from build123d import *

# Parameters (mm, degrees)
SKETCH1_W                = 36
SKETCH1_H                = 22.4
SKETCH1_R                = 1.6
BOSS_EXTRUDE1_DEPTH      = 9.35
FILLET1_R                = 5
SKETCH2_R                = 3.5
BOSS_EXTRUDE2_DEPTH      = 0.3
BOSS_EXTRUDE4_START      = -0.3
BOSS_EXTRUDE4_DEPTH      = 8.4
M3_CLEARANCE_HOLE1_D     = 3.4
M3_CLEARANCE_HOLE1_DEPTH = 8.0000094
M3_CLEARANCE_HOLE1_TIP   = 1.021463052
BOSS_EXTRUDE5_DEPTH      = 9.5
BOSS_EXTRUDE6_DEPTH      = 23
BOSS_EXTRUDE7_DEPTH      = 13.5
SKETCH11_W               = 3.9
SKETCH11_H               = 13.4
CUT_EXTRUDE1_DEPTH       = 5
SKETCH13_W               = 4.8
SKETCH13_H               = 5
SKETCH13_R               = 1.5
BOSS_EXTRUDE8_DEPTH      = 2.75
FILLET2_R                = 1


with BuildPart() as part:
    # Sketch1 → Boss-Extrude1 (new, symmetric)
    with BuildSketch(Plane(origin=(0, 0, 0), x_dir=(1, 0, 0), z_dir=(0, 1, 0))):
        Rectangle(SKETCH1_W, SKETCH1_H)
        with Locations(Location((-13, 8.75, 0), (0, 0, 270))):
            Circle(SKETCH1_R, mode=Mode.SUBTRACT)
        with Locations(Location((-13, -8.75, 0), (0, 0, 270))):
            Circle(SKETCH1_R, mode=Mode.SUBTRACT)
    extrude(amount=BOSS_EXTRUDE1_DEPTH, both=True)

    # Fillet1
    fillet1_edges = [part.edges().sort_by_distance(p)[0] for p in [
        (18, 0, 11.2),
        (18, 0, -11.2),
    ]]
    fillet(fillet1_edges, radius=FILLET1_R)

    # Sketch2 → Boss-Extrude2 (add)
    with BuildSketch(Plane(origin=(0, 9.35, 0), x_dir=(1, 0, 0), z_dir=(0, 1, 0))):
        with Locations(Location((6.7, 0, 0), (0, 0, 90))):
            Circle(SKETCH2_R)
    extrude(amount=BOSS_EXTRUDE2_DEPTH)

    # Sketch3 → Boss-Extrude4 (add)
    with BuildSketch(Plane(origin=(0, 9.65, 0), x_dir=(1, 0, 0), z_dir=(0, 1, 0)).offset(BOSS_EXTRUDE4_START)):
        with BuildLine():
            ThreePointArc((4.716700981, 1.905), (4.148865713, 1.026749165), (3.95, 0))
            Line((3.95, 0), (9.45, 0))
            ThreePointArc((9.45, 0), (9.251134287, 1.026749165), (8.683299019, 1.905))
            Line((8.683299019, 1.905), (4.716700981, 1.905))
        make_face()
        with BuildLine():
            Line((9.45, 0), (3.95, 0))
            ThreePointArc((3.95, 0), (4.148865713, -1.026749165), (4.716700981, -1.905))
            Line((4.716700981, -1.905), (8.683299019, -1.905))
            ThreePointArc((8.683299019, -1.905), (9.251134287, -1.026749165), (9.45, 0))
        make_face()
    extrude(amount=BOSS_EXTRUDE4_DEPTH)

    # M3 Clearance Hole1
    with Locations(Plane(origin=(6.7, 17.75, 0), x_dir=(0, 0, 1), z_dir=(0, 1, 0))):
        with Locations((0, 0)):
            Hole(M3_CLEARANCE_HOLE1_D / 2, depth=M3_CLEARANCE_HOLE1_DEPTH)
            with Locations((0, 0, -(M3_CLEARANCE_HOLE1_DEPTH + M3_CLEARANCE_HOLE1_TIP / 2))):  # 118° drill point
                Cone(0, M3_CLEARANCE_HOLE1_D / 2, M3_CLEARANCE_HOLE1_TIP, mode=Mode.SUBTRACT)

    # Sketch7 → Boss-Extrude5 (add)
    with BuildSketch(Plane.ZY.offset(18)):
        with BuildLine():
            ThreePointArc((-11.2, -2.901648127), (-10.306415682, -6.352188829), (-8.378242386, -9.35))
            Line((-8.378242386, -9.35), (8.378242386, -9.35))
            ThreePointArc((8.378242386, -9.35), (10.306415682, -6.352188829), (11.2, -2.901648127))
            Line((11.2, -2.901648127), (11.2, -0.782686117))
            ThreePointArc((11.2, -0.782686117), (9.493833141, 4.193529382), (5.711776998, 7.85))
            Line((5.711776998, 7.85), (-5.711776998, 7.85))
            ThreePointArc((-5.711776998, 7.85), (-9.493833141, 4.193529382), (-11.2, -0.782686117))
            Line((-11.2, -0.782686117), (-11.2, -2.901648127))
        make_face()
    extrude(amount=BOSS_EXTRUDE5_DEPTH)

    # Sketch8 → Boss-Extrude6 (add)
    with BuildSketch(Plane.ZY.offset(27.5)):
        with BuildLine():
            Line((12.7, -2.97021854), (12.7, -0.714115705))
            ThreePointArc((12.7, -0.714115705), (10.665331767, 5.144477158), (6.107200268, 9.35))
            Line((6.107200268, 9.35), (-6.107200268, 9.35))
            ThreePointArc((-6.107200268, 9.35), (-10.665331767, 5.144477158), (-12.7, -0.714115705))
            Line((-12.7, -0.714115705), (-12.7, -2.97021854))
            ThreePointArc((-12.7, -2.97021854), (-11.554180407, -7.233216661), (-9.023383337, -10.85))
            Line((-9.023383337, -10.85), (9.023383337, -10.85))
            ThreePointArc((9.023383337, -10.85), (11.554180407, -7.233216661), (12.7, -2.97021854))
        make_face()
    extrude(amount=BOSS_EXTRUDE6_DEPTH)

    # Sketch9 → Boss-Extrude7 (add)
    with BuildSketch(Plane.ZY.offset(57.000000114)):
        with BuildLine():
            Line((-8.4, -1.842167122), (-8.4, -6.489747138))
            ThreePointArc((-8.4, -6.489747138), (0, -11.442167122), (8.4, -6.489747138))
            Line((8.4, -6.489747138), (8.4, -1.842167122))
            Line((8.4, -1.842167122), (-8.4, -1.842167122))
        make_face()
        with BuildLine():
            ThreePointArc((8.4, -6.489747138), (0, -11.442167122), (-8.4, -6.489747138))
            Line((-8.4, -6.489747138), (-8.4, -18.454988755))
            Line((-8.4, -18.454988755), (8.4, -18.454988755))
            Line((8.4, -18.454988755), (8.4, -6.489747138))
        make_face()
        with BuildLine():
            Line((3.375, 7.145011245), (-3.375, 7.145011245))
            ThreePointArc((-3.375, 7.145011245), (-9.007736413, 1.477574541), (-8.4, -6.489747138))
            Line((-8.4, -6.489747138), (-8.4, -1.842167122))
            Line((-8.4, -1.842167122), (8.4, -1.842167122))
            Line((8.4, -1.842167122), (8.4, -6.489747138))
            ThreePointArc((8.4, -6.489747138), (9.295160031, -4.242167122), (9.6, -1.842167122))
            ThreePointArc((9.6, -1.842167122), (7.891767863, 3.624093025), (3.375, 7.145011245))
        make_face()
    extrude(amount=-BOSS_EXTRUDE7_DEPTH)

    # Sketch11 → Cut-Extrude1 (cut)
    with BuildSketch(Plane.XZ.offset(18.454988755)):
        with Locations((-48.450000114, 0)):
            Rectangle(SKETCH11_W, SKETCH11_H)
    extrude(amount=-CUT_EXTRUDE1_DEPTH, mode=Mode.SUBTRACT)

    # Sketch13 → Boss-Extrude8 (add)
    with BuildSketch(Plane(origin=(0, -2.149999922, 0), x_dir=(1, 0, 0), z_dir=(0, 1, 0))):
        with Locations((20.4, 0)):
            Rectangle(SKETCH13_W, SKETCH13_H)
        with Locations(Location((20.4, 0, 0), (0, 0, 270))):
            Circle(SKETCH13_R, mode=Mode.SUBTRACT)
    extrude(amount=BOSS_EXTRUDE8_DEPTH)

    # Fillet2
    fillet2_edges = [part.edges().sort_by_distance(p)[0] for p in [
        (18, -0.774999922, -2.5),
        (18, -0.774999922, 2.5),
    ]]
    fillet(fillet2_edges, radius=FILLET2_R)


solid = part.part
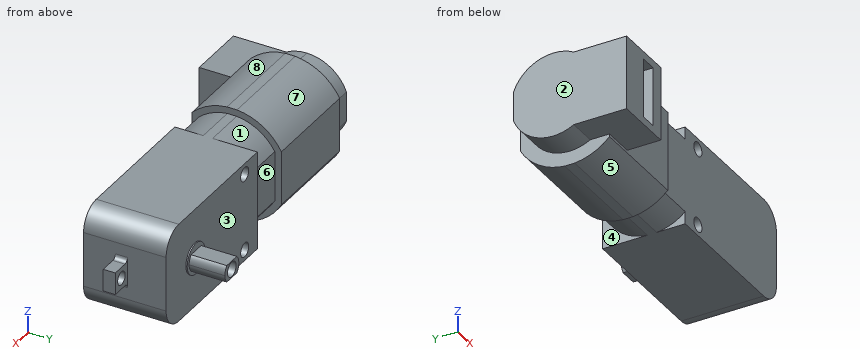
For this review, take the finished solid that the model builds, in its own axes (mm). Face numbers are marked on the shaded views. A direction names the side the tool comes from. Coordinates: 2 decimals unless noted, no trailing zeros. Order: outer loops, then holes, each group sorted by start corner. A loop starts at its lowest first (then second) coordinate and runs counter-clockwise, first axis right, second up. Notation, with made-up numbers: (89, 85) - (93, 85) arc R24 cw to (93, 120) - close; hole circle Ø8 at (79, 82.5). An arc over 180 degrees is marked (long way). Use one line per item in the form item = value.
Q1. Consider section D-D (y = 11). Give the boundary of the cut face in (x, z) (3 decimals), then the cut area to 3 significant figures.
Checked values:
outline = (4.717, -1.905) - (8.683, -1.905) arc R2.75 ccw to (8.683, 1.905) - (4.717, 1.905) arc R2.75 ccw to start; hole circle Ø3.4 at (6.7, 0)
area = 10.1 mm2
Q2. Draft analysis for pull direction X (two halves, no side actions). For the marked faces 1, 2 and 3, state which applies: +X half, -X half, draft (parallel to the pull), parting line (faces both ways), or undercut.
Checked values:
face_1 = undercut
face_2 = -X half
face_3 = draft
Q3. For the marked faces 4, 5, 6, 7 and 8, list the 3-axis set-ups (+Z, -Z, +X, -X, +Y, -Y) from which the entire face can be reached by the end or side of a thin tool; tool diameter is ignored.
Checked values:
face_4 = +Y
face_5 = -Z, -X, -Y
face_6 = +Z, -Z, +Y
face_7 = +Z, -X, +Y
face_8 = +Z, -X, -Y
Q4. For P1, Ø4, axis at x = -13, z = -8.75, coming from the -Y side; P2, Ø1, axis at x = -6.5, z = 2, coming from the +Y side; P3, Ø1, axis at x = -15.5, y = 6, coming from the -Z side, all flat-tipped, find the tip position at first contact; note any pin that passes through.
Checked values:
P1 = -9.35
P2 = 9.35
P3 = -11.2
Q5. Consider section C-C (y = 4). Give the boundary of the cut face in (x, z).
Checked values:
outline = (-57, -7.62) - (-50.5, -7.62) - (-50.5, -11.33) - (-27.5, -11.33) - (-27.5, -9.61) - (-18, -9.61) - (-18, -11.2) - (13, -11.2) arc R5 ccw to (18, -6.2) - (18, 6.2) arc R5 ccw to (13, 11.2) - (-18, 11.2) - (-18, 9.61) - (-27.5, 9.61) - (-27.5, 11.33) - (-50.5, 11.33) - (-50.5, 7.62) - (-57, 7.62) - close; hole circle Ø3.2 at (-13, -8.75); hole circle Ø3.2 at (-13, 8.75)
Q6. Consider section B-B (x = -24). Give the boundary of the cut face in (y, z).
Checked values:
outline = (-9.35, -8.38) arc R11.25 ccw to (-2.9, -11.2) - (-0.78, -11.2) arc R11.25 ccw to (7.85, -5.71) - (7.85, 5.71) arc R11.25 ccw to (-0.78, 11.2) - (-2.9, 11.2) arc R11.25 ccw to (-9.35, 8.38) - close
Q7. Consider section A-A (y = -14.5). Give the boundary of the cut face in (x, z), then the cut area to 3 significant figures.
Checked values:
outline = (-57, -8.4) - (-43.5, -8.4) - (-43.5, 8.4) - (-57, 8.4) - close; hole (-50.4, -6.7) - (-46.5, -6.7) - (-46.5, 6.7) - (-50.4, 6.7) - close
area = 175 mm2
Q8. For probe 1 along X at (y, z) = (-0.5, 0); probe 2 along X at (y, z) = (4, 1); probe 3 along Z at (x, y) = (-8, -1), list the stretches that pass through material, from the lowest coordinate up. Write a range as from..to.
Checked values:
probe_1 = -57..18.9, 21.9..22.8
probe_2 = -57..18
probe_3 = -11.2..11.2
